Build history of the part. All positions in model axes, mm. Round coordinates to 2 decimals unless told otherwise and drop trailing zeros. Loops run counter-clockwise (first coordinate to the right, second up) from the corner with the lowest first, then second, coordinate; pieces in that order, holes last.
Autodesk Inventor part; units mm, degrees
ref_plane "YZ Plane" through (0, 0, 0) normal (1, 0, 0) x (0, 1, 0)
ref_plane "XZ Plane" through (0, 0, 0) normal (0, 1, 0) x (-1, 0, 0)
ref_plane "XY Plane" through (0, 0, 0) normal (0, 0, 1) x (1, 0, 0)
sketch "Skizze1" plane through (0, 0, 0) normal (0, 0, 1) x (1, 0, 0)
  line L0 (-1.4434, 2.5) -> (1.4434, 2.5)
  line L1 (1.4434, 2.5) -> (2.8868, 0)
  line L2 (2.8868, 0) -> (1.4434, -2.5)
  line L3 (1.4434, -2.5) -> (-1.4434, -2.5)
  line L4 (-1.4434, -2.5) -> (-2.8868, 0)
  line L5 (-2.8868, 0) -> (-1.4434, 2.5)
  point P0 (0, 0)
  point P1 (0, 0)
  point P2 (0, 2.5)
  point P3 (0, -2.5)
  dimension "d3" = 120
  dimension "d4" = 120
  dimension "d5" = 120
  dimension "d6" = 5
extrude "Extrusion1" add sketch "Skizze1" along normal blind 10
sketch "Skizze2" plane through (0, 0, 10) normal (0, 0, 1) x (1, 0, 0)
  point P0 (0, 0)
  point P1 (0, 0)
hole "Bohrung1" at (0, 0, 10) direction (0, 0, -1) diameter 2.5 end through all
thread "Gewinde1"
properties part number "10mm_Innengewinde"
(1) Pull direction X, two halves, no side cores. Call faces 1 (the face through (2.155, 1.267, 4.93)), 2 (the face through (1.22, 0.27, 4.93)), 3 (the face through (-2.155, -1.267, 4.93)): +X half, -X half, draft (parallel to the pull), parting line (faces both ways), or undercut.
Responses:
face 1: +X half
face 2: undercut
face 3: -X half
(2) Probe line 1 (Y direction, x = 0, z = 7.25); line 2 (Y direction, x = -0.65, z = 2); line 3 (X direction, y = -2.2, z = 4). List the from-to ranges inside material, lowest first.
Responses:
line 1: y = -2.5 to -1.25, 1.25 to 2.5
line 2: y = -2.5 to -1.07, 1.07 to 2.5
line 3: x = -1.62 to 1.62
(3) Slice it at C-C on y = -0.2. List the corners of the cut face in (x, z).
Responses:
outline: (-2.77, 0) - (-1.23, 0) - (-1.23, 10) - (-2.77, 10) - close; (1.23, 0) - (2.77, 0) - (2.77, 10) - (1.23, 10) - close
(4) Pin check, flat tip, straight feed: P1, Ø1.5, axis at x = 1.5, y = -2, coming from the -Z side. Stop position of the tip, or through.
Responses:
P1: stops at z = 0
(5) Slice it at B-B on z = 4.75. List the corners of the cut face in (x, y).
Responses:
outline: (-2.89, 0) - (-1.44, -2.5) - (1.44, -2.5) - (2.89, 0) - (1.44, 2.5) - (-1.44, 2.5) - close; hole circle Ø2.5 at (0, 0)
(6) Slice it at A-A on x = 0. List the corners of the cut face in (y, z), plus the area to 3 significant figures.
Responses:
outline: (-2.5, 0) - (-1.25, 0) - (-1.25, 10) - (-2.5, 10) - close; (1.25, 0) - (2.5, 0) - (2.5, 10) - (1.25, 10) - close
area: 25.0 mm2
(7) Slice it at D-D on x = 1.7. List the corners of the cut face in (y, z).
Responses:
outline: (-2.06, 0) - (2.06, 0) - (2.06, 10) - (-2.06, 10) - close
